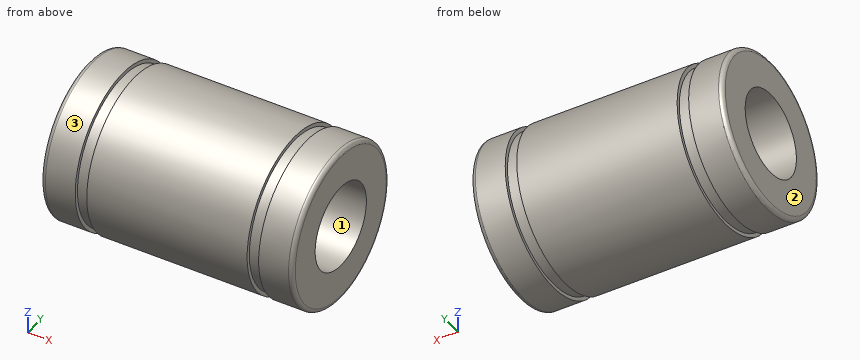
from build123d import *


with BuildPart() as part:
    # Sketch1 → Revolve1 (revolve)
    with BuildSketch(Plane.XY):
        with BuildLine():
            Line((0, 7.1), (0, 4))
            Line((0, 4), (24, 4))
            Line((24, 4), (24, 7.1))
            ThreePointArc((24, 7.1), (23.882842712, 7.382842712), (23.6, 7.5))
            Line((23.6, 7.5), (20.75, 7.5))
            Line((20.75, 7.5), (20.75, 7.15))
            Line((20.75, 7.15), (19.65, 7.15))
            Line((19.65, 7.15), (19.65, 7.5))
            Line((19.65, 7.5), (4.35, 7.5))
            Line((4.35, 7.5), (4.35, 7.15))
            Line((4.35, 7.15), (3.25, 7.15))
            Line((3.25, 7.15), (3.25, 7.5))
            Line((3.25, 7.5), (0.4, 7.5))
            ThreePointArc((0.4, 7.5), (0.117157288, 7.382842712), (0, 7.1))
        make_face()
    revolve(axis=Axis((-0.001253994, 0, 0), (1, 0, 0)))


solid = part.part
Check sheet for the modelled part. Datum: model origin and axes. Units: mm. Face numbers are marked on the shaded views. Give positions to 0.01 mm unless a question says otherwise; leave off trailing zeros. Loops run counter-clockwise (first coordinate to the right, second up) from the corner with the lowest first, then second, coordinate; pieces in that order, holes last. Notation, with made-up numbers: M 49,6 L 79,6 A26 cw 79,23 Z; hole C 18,46 d4. An arc over 180 degrees is marked long. Answer as a JSON object with one key per item and string values. Group by question number.
Q1. Release check for a two-part mould opening along Z. For the marked faces 1, 2 and 3 record: released by +Z, released by -Z, zero draft, split by the parting line, or undercut.
Q2. Cross-section at D-D on x = 9. Record the cut outline in (y, z), then the cut area to 3 significant figures.
Q3. Go/stop test with a flat-tipped pin: P1, Ø6, axis at x = 15, z = -4, coming from the -Y side. Record where the tip stops, or that it passes through.
Q4. Cross-section at C-C on x = 4. Record the cut outline in (y, z), then the cut area to 3 significant figures.
Q5. Cross-section at A-A on y = 0. Record the cut outline in (x, z).
Q6. Material ranges on line 1 along Z through (x, y) = (19, 0); line 2 along Y through (x, z) = (20.5, -3.25); line 3 along Z through (x, y) = (22.5, -1), recorded low to high. Write a range as [from, to].
Evaluation:
{
 "1": {"face 1": "undercut", "face 2": "zero draft", "face 3": "split by the parting line"},
 "2": {"outline": "C 0,0 d15; hole C 0,0 d8", "area": "126 mm2"},
 "3": {"P1": "stops at y = -7.43"},
 "4": {"outline": "C 0,0 d14.3; hole C 0,0 d8", "area": "110 mm2"},
 "5": {"outline": "M 0,-7.1 A0.4 ccw 0.4,-7.5 L 3.25,-7.5 L 3.25,-7.15 L 4.35,-7.15 L 4.35,-7.5 L 19.65,-7.5 L 19.65,-7.15 L 20.75,-7.15 L 20.75,-7.5 L 23.6,-7.5 A0.4 ccw 24,-7.1 L 24,-4 L 0,-4 Z; M 0,4 L 24,4 L 24,7.1 A0.4 ccw 23.6,7.5 L 20.75,7.5 L 20.75,7.15 L 19.65,7.15 L 19.65,7.5 L 4.35,7.5 L 4.35,7.15 L 3.25,7.15 L 3.25,7.5 L 0.4,7.5 A0.4 ccw 0,7.1 Z"},
 "6": {"line 1": "z = [-7.5, -4], [4, 7.5]", "line 2": "y = [-6.37, -2.33], [2.33, 6.37]", "line 3": "z = [-7.43, -3.87], [3.87, 7.43]"}
}
